Check sheet for the drawn part. Datum: minimum x, y, z corner. Units: mm. A direction names the side the tool comes from. Coordinates: 2 decimals unless noted, no trailing zeros. Write each loop counter-clockwise with the first axis right and the second up, starting at its lowest first coordinate (ties: lowest second). Pieces come first, ordered by that corner, then holes. Notation, with made-up numbers: (10.25, 43.25) - (44.25, 43.25) arc R9 ccw to (44.25, 51.25) - close; hole circle Ø9 at (46.25, 46.5). An arc over 180 degrees is marked (long way). Use one line per item in the form item = value. Start each with the question number.
1. Tool access check on the marked faces 1 and 2. Record the directions out of +Z, -Z, +X, -X, +Y, -Y that give a thin tool (end or side, any length) a straight path to the whole face; none if there is none.
2. Draft check along X on the marked faces 3, 4, 5 and 6. Enter one of: +X half, -X half, draft (parallel to the pull), parting line (faces both ways), or undercut.
3. Cross-section at B-B on y = 9. Record the boundary of the cut face in (x, z).
4. Cross-section at C-C on z = 52. Record the boundary of the cut face in (x, y).
5. Cross-section at D-D on x = 19.5. Record the boundary of the cut face in (y, z).
6. Go/stop test with flat-tipped pins: pin 1 Ø6 at (x, y) = (66, 15) entering from -Z; pin 2 Ø4 at (x, z) = (8.29, 62.305) entering from +Y. Record where each tip stops, or that it passes through.
7. Scan lines: line 1 along Z through (x, y) = (16, 9); line 2 along X through (y, z) = (10.5, 27); line 3 along Y through (x, z) = (5, 40.5). Record each from-to range of solid material in increasing order.
8. Cross-section at A-A on x = 8.29. Record the boundary of the cut face in (y, z).
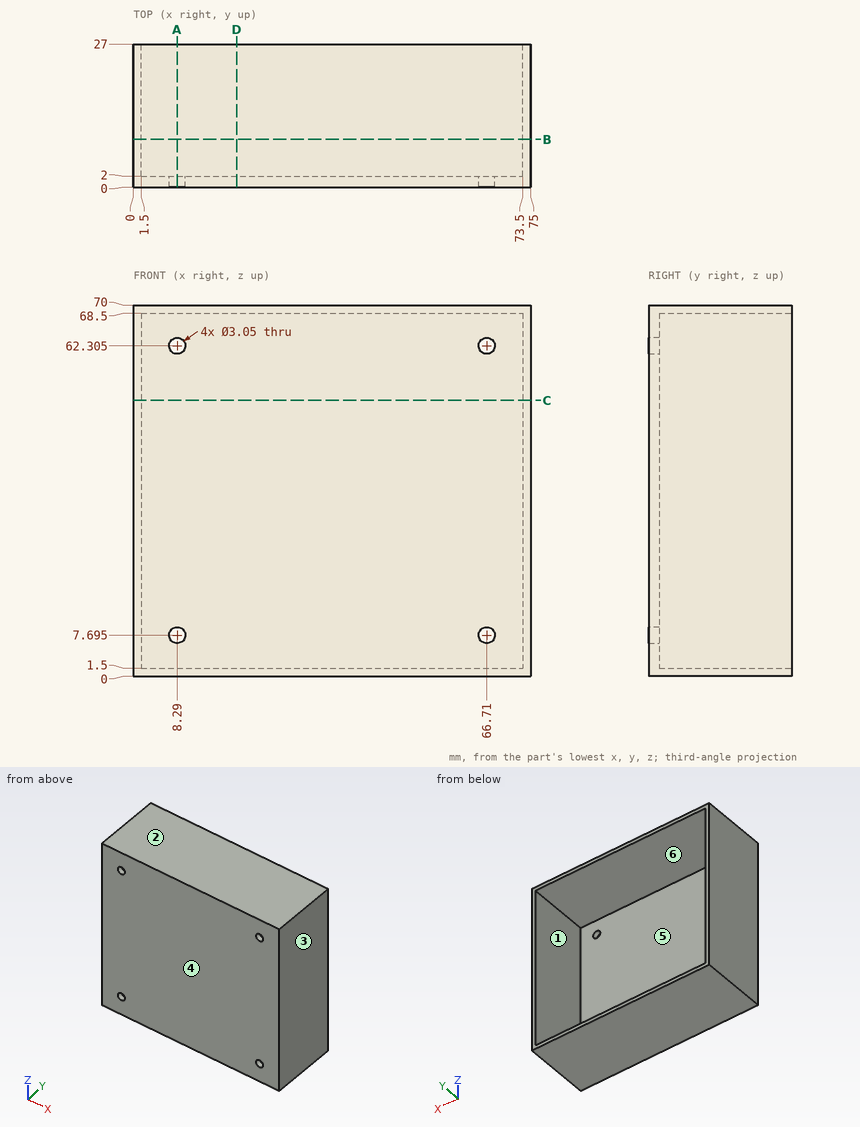
Final values:
q1.face_1 = +Y
q1.face_2 = +Z, +X, -X, +Y, -Y
q2.face_3 = +X half
q2.face_4 = draft
q2.face_5 = undercut
q2.face_6 = undercut
q3.outline = (0, 0) - (75, 0) - (75, 70) - (0, 70) - close; hole (1.5, 1.5) - (73.5, 1.5) - (73.5, 68.5) - (1.5, 68.5) - close
q4.outline = (0, 0) - (75, 0) - (75, 27) - (73.5, 27) - (73.5, 2) - (1.5, 2) - (1.5, 27) - (0, 27) - close
q5.outline = (0, 0) - (27, 0) - (27, 1.5) - (2, 1.5) - (2, 68.5) - (27, 68.5) - (27, 70) - (0, 70) - close
q6.pin_1 = 0
q6.pin_2 = 2
q7.line_1 = 0 to 1.5, 68.5 to 70
q7.line_2 = 0 to 1.5, 73.5 to 75
q7.line_3 = 0 to 2
q8.outline = (0, 0) - (27, 0) - (27, 1.5) - (2, 1.5) - (2, 6.17) - (0, 6.17) - close; (0, 9.22) - (2, 9.22) - (2, 60.78) - (0, 60.78) - close; (0, 63.83) - (2, 63.83) - (2, 68.5) - (27, 68.5) - (27, 70) - (0, 70) - close
